The listing builds one solid part. Answer for the finished solid, in the listing's coordinates (mm). A direction names the side the tool comes from. Round coordinates to 2 decimals unless told otherwise and drop trailing zeros. Write each loop counter-clockwise with the first axis right and the second up, starting at its lowest first coordinate (ties: lowest second). Pieces come first, ordered by that corner, then holes. Notation, with made-up numbers: (13, 23.5) - (72, 23.5) arc R15 ccw to (72, 49.5) - close; hole circle Ø8 at (65.25, 82). An arc over 180 degrees is marked (long way). Answer as CSV lines item,"result". Start each with the question number.
Item 1: Which of the six approach directions +Z, -Z, +X, -X, +Y, -Y give full straight-line access (tool end or side, diameter ignored) to faces 1 (the cylindrical face through (-9.183, 22.93, -13.898)), 2 (the flat face through (20, 14, 0)), 3 (the flat face through (9, 18, -13))?
Item 2: A cutting plane is placed at A-A on y = 11. Determine the outline of the cut face in (x, z), and give its area (3 significant figures).
Item 3: A cutting plane is placed at C-C on z = 16. Determine the outline of the cut face in (x, y).
Item 4: A cutting plane is placed at D-D on y = 25.75. State how many separate pieces and enclosed holes the cut face has, and give its area (3 significant figures).
Item 5: Straight lines are drawn through the part: line 1 along X through (y, z) = (6, 0); line 2 along Z through (x, y) = (-5, 8.75); line 3 along X through (y, z) = (21, 16). For each, find the intervals that lie inside material, in ascending order. Write a range as [from, to].
Item 6: Flat-ended cylindrical pins translate along their axes: pin 1 (3 mm diameter, centred on x = 10, z = 9, fed in from +Y); pin 2 (3 mm diameter, centred on x = -10, z = -13, fed in from -Y). Find the tip coordinate at first contact, or state that the pin passes through.
Item 7: A cutting plane is placed at B-B on z = 0. Determine the outline of the cut face in (x, y), and give its area (3 significant figures).
Item 8: For a pull along Z with two mould halves and no side action, classify faces 4 (the flat face through (0, 28, 0)), 5 (the cylindrical face through (17.735, 14.196, -16.228)), 6 (the flat face through (0, 14, 20)) as pulls with the +Z half, pulls with the -Z half, needs draft (parallel to the pull), parting line crosses it, or undercut.
```python
from build123d import *

# Parameters (mm, degrees)
EXTRUDE_1_DEPTH          = 28
SKETCH_2_R               = 1.75
CUT_EXTRUDE_1_DEPTH      = 40.799497484
SKETCH_3_R               = 19
SKETCH_3_R_2             = 10
CUT_EXTRUDE_2_DEPTH      = 40.799497484
EXTRUDE_2_DEPTH          = 10
PATTERN_START            = 18
PATTERN_CIRCULAR_1_DEPTH = 10


# Read off the part's stored shape, not the designer's step: the pattern circular step
with BuildPart() as part:
    # Sketch 1 → Extrude 1 (new body)
    with BuildSketch(Plane(origin=(0, 0, 0), x_dir=(1, 0, 0), z_dir=(0, 1, 0))):
        with BuildLine():
            Line((-15, 20), (15, 20))
            ThreePointArc((15, 20), (18.535533906, 18.535533906), (20, 15))
            Line((20, 15), (20, -15))
            ThreePointArc((20, -15), (18.535533906, -18.535533906), (15, -20))
            Line((15, -20), (-15, -20))
            ThreePointArc((-15, -20), (-18.535533906, -18.535533906), (-20, -15))
            Line((-20, -15), (-20, 15))
            ThreePointArc((-20, 15), (-18.535533906, 18.535533906), (-15, 20))
        make_face()
    extrude(amount=EXTRUDE_1_DEPTH)

    # Sketch 2 → Cut-Extrude 1 (cut, through all)
    with BuildSketch(Plane(origin=(0, 28, 0), x_dir=(1, 0, 0), z_dir=(0, 1, 0))):
        with Locations(Location((-16, 16, 0), (0, 0, 270))):
            Circle(SKETCH_2_R)
        with Locations(Location((16, 16, 0), (0, 0, 270))):
            Circle(SKETCH_2_R)
        with Locations(Location((16, -16, 0), (0, 0, 270))):
            Circle(SKETCH_2_R)
        with Locations(Location((-16, -16, 0), (0, 0, 270))):
            Circle(SKETCH_2_R)
    extrude(amount=-CUT_EXTRUDE_1_DEPTH, mode=Mode.SUBTRACT)

    # Sketch 3 → Cut-Extrude 2 (cut, through all)
    with BuildSketch(Plane(origin=(0, 28, 0), x_dir=(1, 0, 0), z_dir=(0, 1, 0))):
        with Locations(Location((0, 0, 0), (0, 0, 270))):
            Circle(SKETCH_3_R)
        with Locations(Location((0, 0, 0), (0, 0, 270))):
            Circle(SKETCH_3_R_2, mode=Mode.SUBTRACT)
    extrude(amount=-CUT_EXTRUDE_2_DEPTH, mode=Mode.SUBTRACT)


with BuildPart() as cut_extrude_2_piece_1:
    # of the separate pieces the step leaves, piece 1, a body of its own (cut_extrude_2_pieces)
    add(part.part.solids().sort_by_distance((-15, 0, -20))[0])



with BuildPart() as cut_extrude_2_piece_2:
    # of the separate pieces the step leaves, piece 2, a body of its own (cut_extrude_2_pieces)
    add(part.part.solids().sort_by_distance((0, 0, 10))[0])


with BuildPart() as cut_extrude_2_piece_1_1:
    add(cut_extrude_2_piece_1.part)

    add(cut_extrude_2_piece_2.part)  # Extrude 2 merges Cut-Extrude 2 piece 2
    # Sketch 4 → Extrude 2 (add)
    with BuildSketch(Plane(origin=(0, 28, 0), x_dir=(1, 0, 0), z_dir=(0, 1, 0))):
        with BuildLine():
            Line((0, 20), (0, 19))
            ThreePointArc((0, 19), (8.809946394, 10.190053606), (0, 1.380107213))
            Line((0, 1.380107213), (0, 0))
            ThreePointArc((0, 0), (10, 10), (0, 20))
        make_face()
    extrude(amount=-EXTRUDE_2_DEPTH)

    # Pattern Circular 1 outline → Pattern Circular 1 (add)
    with BuildSketch(Plane(origin=(0, 0, 0), x_dir=(1, 0, 0), z_dir=(0, 1, 0)).offset(PATTERN_START)):
        with BuildLine():
            ThreePointArc((-1.43801989, 9.896064814), (-0.720885519, 9.973982358), (0, 10))
            ThreePointArc((0, 10), (-5.537755039, 14.5), (-12.665384489, 14.162910568))
            ThreePointArc((-12.665384489, 14.162910568), (-14.745417919, 11.982180536), (-16.454482672, 9.5))
            ThreePointArc((-16.454482672, 9.5), (-9.057130134, 13.90191043), (-1.43801989, 9.896064814))
        make_face()
        with BuildLine():
            ThreePointArc((18.598132588, 3.887089432), (17.749581696, 6.778816239), (16.454482672, 9.5))
            ThreePointArc((16.454482672, 9.5), (16.56797266, 0.892749566), (9.289253471, -3.702670651))
            ThreePointArc((9.289253471, -3.702670651), (8.998164858, -4.362686006), (8.660254038, -5))
            ThreePointArc((8.660254038, -5), (15.326245874, -2.454163457), (18.598132588, 3.887089432))
        make_face()
        with BuildLine():
            ThreePointArc((-9.289253471, 3.702670651), (-8.998164858, 4.362686006), (-8.660254038, 5))
            ThreePointArc((-8.660254038, 5), (-15.326245874, 2.454163457), (-18.598132588, -3.887089432))
            ThreePointArc((-18.598132588, -3.887089432), (-17.749581696, -6.778816239), (-16.454482672, -9.5))
            ThreePointArc((-16.454482672, -9.5), (-16.56797266, -0.892749566), (-9.289253471, 3.702670651))
        make_face()
        with BuildLine():
            ThreePointArc((16.454482672, -9.5), (9.057130134, -13.90191043), (1.43801989, -9.896064814))
            ThreePointArc((1.43801989, -9.896064814), (0.720885519, -9.973982358), (0, -10))
            ThreePointArc((0, -10), (5.537755039, -14.5), (12.665384489, -14.162910568))
            ThreePointArc((12.665384489, -14.162910568), (14.745417919, -11.982180536), (16.454482672, -9.5))
        make_face()
        with BuildLine():
            ThreePointArc((-7.851233581, -6.193394163), (-8.277279339, -5.611296352), (-8.660254038, -5))
            ThreePointArc((-8.660254038, -5), (-9.788490836, -12.045836544), (-5.932748098, -18.05))
            ThreePointArc((-5.932748098, -18.05), (-3.004163777, -18.760996775), (0, -19))
            ThreePointArc((0, -19), (-7.510842526, -14.794659996), (-7.851233581, -6.193394163))
        make_face()
    extrude(amount=PATTERN_CIRCULAR_1_DEPTH)


solid = cut_extrude_2_piece_1_1.part
```
Geometry says:
1,face 1,"+Y, -Y"
1,face 2,"+Z, -Z, +X, +Y, -Y"
1,face 3,"-Y"
2,outline,"(-20, -15) arc R5 ccw to (-15, -20) - (15, -20) arc R5 ccw to (20, -15) - (20, 15) arc R5 ccw to (15, 20) - (-15, 20) arc R5 ccw to (-20, 15) - close; circle Ø20 at (0, 0); hole circle Ø38 at (0, 0); hole circle Ø3.5 at (-16, -16); hole circle Ø3.5 at (-16, 16); hole circle Ø3.5 at (16, -16); hole circle Ø3.5 at (16, 16)"
2,area,"720 mm^2"
3,outline,"(-19.9, 0) - (-17.75, 0) - (-17.75, 28) - (-19.9, 28) - close; (-14.25, 0) - (-10.25, 0) - (-10.25, 28) - (-14.25, 28) - close; (-8, 18) - (-6.62, 18) - (-6.62, 28) - (-8, 28) - close; (10.25, 0) - (14.25, 0) - (14.25, 28) - (10.25, 28) - close; (17.75, 0) - (19.9, 0) - (19.9, 28) - (17.75, 28) - close"
4,separate pieces,"1"
4,enclosed holes,"10"
4,area,"825 mm^2"
5,line 1,"x = [-20, -19], [-10, 10], [19, 20]"
5,line 2,"z = [-20, -18.33], [-8.66, 8.66], [18.33, 20]"
5,line 3,"x = [-19.9, -17.75], [-14.25, -10.25], [-8, -6.62], [10.25, 14.25], [17.75, 19.9]"
6,pin 1,"passes through"
6,pin 2,"stops at y = 18"
7,outline,"(-20, 0) - (-19, 0) - (-19, 28) - (-20, 28) - close; (-17.32, 18) - (-16.01, 18) - (-16.01, 28) - (-17.32, 28) - close; (-10, 0) - (10, 0) - (10, 28) - (-10, 28) - close; (16.01, 18) - (17.32, 18) - (17.32, 28) - (16.01, 28) - close; (19, 0) - (20, 0) - (20, 28) - (19, 28) - close"
7,area,"642 mm^2"
8,face 4,"needs draft"
8,face 5,"undercut"
8,face 6,"pulls with the +Z half"
